from build123d import *

# Parameters (mm, degrees)
F0_W     = 139.7
F0_H     = 69.85
F1_DEPTH = 22.225
F2_W     = 101.6
F2_H     = 34.925
F3_DEPTH = 12.7
F4_W     = 15.875
F4_H     = 19.05
F5_DEPTH = 127


with BuildPart() as f1:
    # F0 (on Front) → F1 (new body)
    with BuildSketch(Plane.XZ):
        Rectangle(F0_W, F0_H)
    extrude(amount=F1_DEPTH)

    # F2 (on face) → F3 (cut)
    with BuildSketch(Plane.XZ.offset(22.225)):
        with Locations((-19.05, 17.4625)):
            Rectangle(F2_W, F2_H)
    extrude(amount=-F3_DEPTH, mode=Mode.SUBTRACT)

    # F4 (on face) → F5 (cut)
    with BuildSketch(Plane.XY.offset(34.925)):
        with Locations((61.9125, -12.7)):
            Rectangle(F4_W, F4_H)
    extrude(amount=-F5_DEPTH, mode=Mode.SUBTRACT)


solid = f1.part
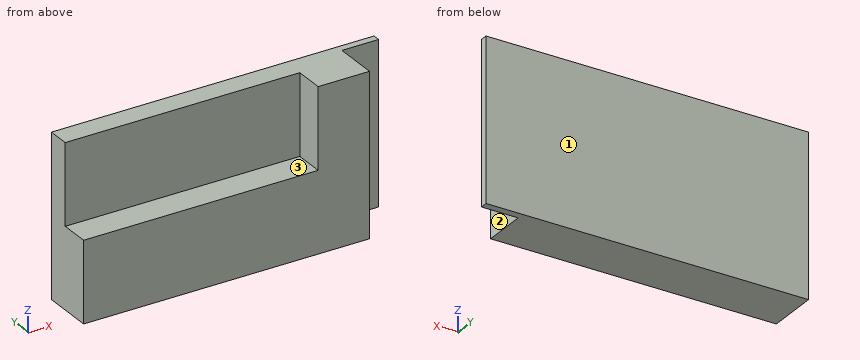
Work out the finished part from the listing and answer in its coordinate system (mm). Face numbers are marked on the shaded views. A direction names the side the tool comes from. Coordinates: 2 decimals unless noted, no trailing zeros. Write each loop counter-clockwise with the first axis right and the second up, starting at its lowest first coordinate (ties: lowest second). Pieces come first, ordered by that corner, then holes. Notation, with made-up numbers: M 75,21.5 L 94,21.5 A9 ccw 94,36.5 Z; hole C 50.5,30 d3. An arc over 180 degrees is marked long. Answer as CSV lines item,"result". Start each with the question number.
Item 1: A tool of negligible diameter and unlimited length cuts with its end or side. For the marked faces 1, 2 and 3, from which of +Z, -Z, +X, -X, +Y, -Y can it reach the whole face along a straight path? Write none if from no direction.
Item 2: Section C-C on x = 25 is taken. Write down the section's boundary in (y, z) (3 decimals).
Item 3: Flat-ended cylindrical pins translate along their axes: P1, Ø1, axis at y = -14.5, z = -21.5, coming from the +X side (3 decimals); P2, Ø6.5, axis at x = -25.5, y = -15.5, coming from the +Z side; P3, Ø5, axis at x = 59, z = 1, coming from the -Y side (3 decimals). Find the tip coordinate at first contact, or state that the pin passes through.
Item 4: Section D-D on y = -5.5 is taken. Write down the section's boundary in (x, z) (3 decimals), and give its area (3 significant figures).
Item 5: Section A-A on y = -13.5 is taken. Write down the section's boundary in (x, z) (3 decimals), and give its area (3 significant figures).
Item 6: Section B-B on z = 10 is taken. Write down the section's boundary in (x, y) (3 decimals).
Item 7: Consider L1, parallel to Y at x = -39.5, z = 31 (3 decimals); L2, parallel to X at y = -13.5, z = -24 (3 decimals); L3, parallel to X at y = -20.5, z = 19 (3 decimals). Determine where each line is inside the solid, lowest interval first.
Checks:
1,face 1,"+Z, -Z, +X, -X, +Y"
1,face 2,"+Z, -Z, +X, -Y"
1,face 3,"+Z, -X, -Y"
2,outline,"M -22.225,-34.925 L 0,-34.925 L 0,34.925 L -9.525,34.925 L -9.525,0 L -22.225,0 Z"
3,P1,"stops at x = 53.975"
3,P2,"stops at z = 0"
3,P3,"stops at y = -3.175"
4,outline,"M -69.85,-34.925 L 53.975,-34.925 L 53.975,34.925 L -69.85,34.925 Z"
4,area,"8,650 mm²"
5,outline,"M -69.85,-34.925 L 53.975,-34.925 L 53.975,34.925 L 31.75,34.925 L 31.75,0 L -69.85,0 Z"
5,area,"5,100 mm²"
6,outline,"M -69.85,-9.525 L 31.75,-9.525 L 31.75,-22.225 L 53.975,-22.225 L 53.975,-3.175 L 69.85,-3.175 L 69.85,0 L -69.85,0 Z"
7,L1,"y = -9.525 to 0"
7,L2,"x = -69.85 to 53.975"
7,L3,"x = 31.75 to 53.975"
